Build history of the part. All positions in model axes, mm. Face numbers are marked on the shaded views. A direction names the side the tool comes from. Round coordinates to 2 decimals unless told otherwise and drop trailing zeros. Loops run counter-clockwise (first coordinate to the right, second up) from the corner with the lowest first, then second, coordinate; pieces in that order, holes last. Notation, with made-up numbers: (44, 63) -> (72, 63) arc R23 cw to (72, 97) -> close; hole circle Ø1 at (27.5, 85). An arc over 180 degrees is marked (long way). Put each result on its own line as item: value. Start each with the question number.
Item 1: Cut at D-D, the plane z = -28. List the corners of the cut face in (x, y), plus the area to 3 significant figures.
Item 2: Pull direction Z, two halves, no side cores. Call the marked faces 3, 4 and 5: +Z half, -Z half, draft (parallel to the pull), parting line (faces both ways), or undercut.
Item 3: Cut at B-B, the plane x = 0. List the corners of the cut face in (y, z).
Item 4: Tool access for the marked faces 1 and 2: list every direction of +Z, -Z, +X, -X, +Y, -Y with a clear straight run to the whole face (end or side of a thin tool).
Item 5: Flat gauge pins, fed straight in: pin 1 Ø5 at (x, y) = (4, 8) entering from +Z; pin 2 Ø0.9 at (x, y) = (28, 4.5) entering from -Z; pin 3 Ø4 at (y, z) = (4, -13.5) entering from -X; pin 4 Ø23 at (x, z) = (0, 0) entering from +Y. Where does each tip first touch, or does it go through?
Item 6: Cut at C-C, the plane y = 3.25. List the corners of the cut face in (x, z), plus the area to 3 significant figures.
Item 7: Cut at A-A, the plane z = 0. List the corners of the cut face in (x, y), plus the area to 3 significant figures.
Item 8: Drill centre lines: probe 1 along X at (y, z) = (1.15, 0); probe 2 along X at (y, z) = (4, -3); probe 3 along Z at (x, y) = (21.5, 4.5). Where is each one in solid material? Low to high. Write a range as [from, to].
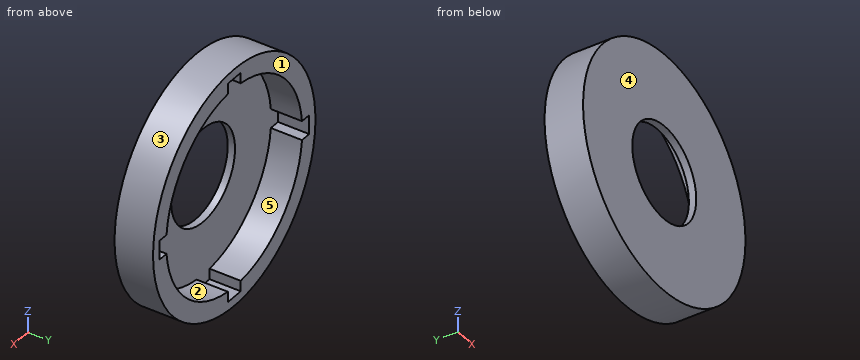
```python
from build123d import *

# Parameters (mm, degrees)
SKETCH1_R           = 32.5
SKETCH1_R_2         = 12.8
BOSS_EXTRUDE1_DEPTH = 2
SKETCH2_R           = 32.5
BOSS_EXTRUDE2_DEPTH = 8.5


with BuildPart() as part:
    # Sketch1 → Boss-Extrude1 (new body)
    with BuildSketch(Plane(origin=(0, 0, 0), x_dir=(1, 0, 0), z_dir=(0, 1, 0))):
        with Locations(Location((0, 0, 0), (0, 0, 270))):
            Circle(SKETCH1_R)
        with Locations(Location((0, 0, 0), (0, 0, 270))):
            Circle(SKETCH1_R_2, mode=Mode.SUBTRACT)
    extrude(amount=BOSS_EXTRUDE1_DEPTH)

    # Sketch2 → Boss-Extrude2 (add)
    with BuildSketch(Plane(origin=(0, 2, 0), x_dir=(1, 0, 0), z_dir=(0, 1, 0))):
        with Locations(Location((0, 0, 0), (0, 0, 270))):
            Circle(SKETCH2_R)
        with BuildLine():
            Line((2.6, -27.125679715), (2.6, -30))
            Line((2.6, -30), (-2.6, -30))
            Line((-2.6, -30), (-2.6, -27.125679715))
            ThreePointArc((-2.6, -27.125679715), (-19.268659787, -19.268659787), (-27.125679715, -2.6))
            Line((-27.125679715, -2.6), (-30, -2.6))
            Line((-30, -2.6), (-30, 2.6))
            Line((-30, 2.6), (-27.125679715, 2.6))
            ThreePointArc((-27.125679715, 2.6), (-19.268659787, 19.268659787), (-2.6, 27.125679715))
            Line((-2.6, 27.125679715), (-2.6, 30))
            Line((-2.6, 30), (2.6, 30))
            Line((2.6, 30), (2.6, 27.125679715))
            ThreePointArc((2.6, 27.125679715), (19.268659787, 19.268659787), (27.125679715, 2.6))
            Line((27.125679715, 2.6), (30, 2.6))
            Line((30, 2.6), (30, -2.6))
            Line((30, -2.6), (27.125679715, -2.6))
            ThreePointArc((27.125679715, -2.6), (19.268659787, -19.268659787), (2.6, -27.125679715))
        make_face(mode=Mode.SUBTRACT)
    extrude(amount=BOSS_EXTRUDE2_DEPTH)


solid = part.part
```
Reply:
1. outline: (-16.5, 0) -> (16.5, 0) -> (16.5, 10.5) -> (2.6, 10.5) -> (2.6, 2) -> (-2.6, 2) -> (-2.6, 10.5) -> (-16.5, 10.5) -> close
1. area: 302 mm^2
2. face 3: parting line
2. face 4: draft
2. face 5: undercut
3. outline: (0, -32.5) -> (10.5, -32.5) -> (10.5, -30) -> (2, -30) -> (2, -12.8) -> (0, -12.8) -> close; (0, 12.8) -> (2, 12.8) -> (2, 30) -> (10.5, 30) -> (10.5, 32.5) -> (0, 32.5) -> close
4. face 1: +Z, -Z, +X, -X, +Y
4. face 2: +Y
5. pin 1: stops at z = 32.47
5. pin 2: stops at z = -17.24
5. pin 3: stops at x = -30.4
5. pin 4: passes through
6. outline: circle Ø65 at (0, 0); hole (-30, -2.6) -> (-27.13, -2.6) arc R27.25 ccw to (-2.6, -27.13) -> (-2.6, -30) -> (2.6, -30) -> (2.6, -27.13) arc R27.25 ccw to (27.13, -2.6) -> (30, -2.6) -> (30, 2.6) -> (27.13, 2.6) arc R27.25 ccw to (2.6, 27.13) -> (2.6, 30) -> (-2.6, 30) -> (-2.6, 27.13) arc R27.25 ccw to (-27.13, 2.6) -> (-30, 2.6) -> close
6. area: 927 mm^2
7. outline: (-32.5, 0) -> (-12.8, 0) -> (-12.8, 2) -> (-30, 2) -> (-30, 10.5) -> (-32.5, 10.5) -> close; (12.8, 0) -> (32.5, 0) -> (32.5, 10.5) -> (30, 10.5) -> (30, 2) -> (12.8, 2) -> close
7. area: 121 mm^2
8. probe 1: x = [-32.5, -12.8], [12.8, 32.5]
8. probe 2: x = [-32.36, -27.08], [27.08, 32.36]
8. probe 3: z = [-24.37, -16.74], [16.74, 24.37]
